Model file for the job. Use its own axes, mm. Face numbers are marked on the shaded views. A direction names the side the tool comes from. Give positions to 0.01 mm unless a question says otherwise; leave off trailing zeros. Loops run counter-clockwise (first coordinate to the right, second up) from the corner with the lowest first, then second, coordinate; pieces in that order, holes last. Notation, with made-up numbers: M -6.5,80.25 L 9.5,80.25 A21 ccw 9.5,116.25 Z; hole C 23,2 d2. An arc over 180 degrees is marked long. Use CSV: the item, a comma, the result in double quotes. Start each with the question number.
(1) Slice it at C-C on y = 46.5. List the corners of the cut face in (x, z).
(2) Two-plate mould, pull along Z, no slides. Class the marked faces 4, 5, 6 and 7: pulls with the +Z half, pulls with the -Z half, needs draft (parallel to the pull), parting line crosses it, or undercut.
(3) Wall check: line 1 along X through (y, z) = (62, -13.5); line 2 along Z through (x, y) = (12, 57); line 3 along Z through (x, y) = (-13, 58). Give the ranges that are in metal, low to high. Write a range as from..to.
(4) Slice it at A-A on z = -13. List the corners of the cut face in (x, y).
(5) Tool access for the marked faces 1, 2 and 3: list every direction of +Z, -Z, +X, -X, +Y, -Y with a clear straight run to the whole face (end or side of a thin tool).
(6) Flat gauge pins, fed straight in: P1, Ø5, axis at x = 12, y = 21, coming from the +Z side; P2, Ø2, axis at x = -8.5, y = 57, coming from the +Z side; P3, Ø8, axis at x = 4, z = 22, coming from the +Y side. Where does each tip first touch, or does it go through?
(7) Slice it at B-B on x = -6. List the corners of the cut face in (y, z).
(8) Slice it at D-D on z = 14. List the corners of the cut face in (x, y), and give its area (3 significant figures).
```python
from build123d import *

# Parameters (mm, degrees)
SKETCH1_R           = 17.5
BOSS_EXTRUDE1_DEPTH = 48
BOSS_EXTRUDE2_DEPTH = 15
BOSS_EXTRUDE3_DEPTH = 20


with BuildPart() as part:
    # Sketch1 → Boss-Extrude1 (new body)
    with BuildSketch(Plane(origin=(0, 0, 0), x_dir=(1, 0, 0), z_dir=(0, 1, 0))):
        Circle(SKETCH1_R)
    extrude(amount=BOSS_EXTRUDE1_DEPTH)

    # Sketch4 → Boss-Extrude2 (add)
    with BuildSketch(Plane.XZ):
        with BuildLine():
            Line((10.25, 23.304288773), (10.25, 16.761190292))
            ThreePointArc((10.25, 16.761190292), (10.701996736, 14.5776924), (11.983695652, 12.75307957))
            ThreePointArc((11.983695652, 12.75307957), (0, 17.5), (-11.983695652, 12.75307957))
            ThreePointArc((-11.983695652, 12.75307957), (-10.701996736, 14.5776924), (-10.25, 16.761190292))
            Line((-10.25, 16.761190292), (-10.25, 23.304288773))
            ThreePointArc((-10.25, 23.304288773), (-9.292662905, 26.079093189), (-6.827982425, 27.673265071))
            ThreePointArc((-6.827982425, 27.673265071), (0, 28.503174274), (6.827982425, 27.673265071))
            ThreePointArc((6.827982425, 27.673265071), (9.292662905, 26.079093189), (10.25, 23.304288773))
        make_face()
    extrude(amount=-BOSS_EXTRUDE2_DEPTH)

    # Sketch6 → Boss-Extrude3 (add)
    with BuildSketch(Plane(origin=(0, 48, 0), x_dir=(1, 0, 0), z_dir=(0, 1, 0))):
        with BuildLine():
            ThreePointArc((11.641553947, -1.685099566), (14.648632583, -1.806960077), (17.329910897, -0.440168758))
            ThreePointArc((17.329910897, -0.440168758), (17.3355, 0), (17.329910897, 0.440168758))
            ThreePointArc((17.329910897, 0.440168758), (14.648632583, 1.806960077), (11.641553947, 1.685099566))
            ThreePointArc((11.641553947, 1.685099566), (11.362069294, 3.044457292), (10.92443124, 4.361437941))
            ThreePointArc((10.92443124, 4.361437941), (13.589567986, 5.759442961), (15.228227462, 8.283758122))
            ThreePointArc((15.228227462, 8.283758122), (15.012983387, 8.66775), (14.788058703, 9.046152775))
            ThreePointArc((14.788058703, 9.046152775), (11.782607909, 8.889189622), (9.239331674, 7.280116005))
            ThreePointArc((9.239331674, 7.280116005), (8.317612002, 8.317612002), (7.280116005, 9.239331674))
            ThreePointArc((7.280116005, 9.239331674), (8.889189622, 11.782607909), (9.046152775, 14.788058703))
            ThreePointArc((9.046152775, 14.788058703), (8.66775, 15.012983387), (8.283758122, 15.228227462))
            ThreePointArc((8.283758122, 15.228227462), (5.759442961, 13.589567986), (4.361437941, 10.92443124))
            ThreePointArc((4.361437941, 10.92443124), (3.044457292, 11.362069294), (1.685099566, 11.641553947))
            ThreePointArc((1.685099566, 11.641553947), (1.806960077, 14.648632583), (0.440168758, 17.329910897))
            ThreePointArc((0.440168758, 17.329910897), (0, 17.3355), (-0.440168758, 17.329910897))
            ThreePointArc((-0.440168758, 17.329910897), (-1.806960077, 14.648632583), (-1.685099566, 11.641553947))
            ThreePointArc((-1.685099566, 11.641553947), (-3.044457292, 11.362069294), (-4.361437941, 10.92443124))
            ThreePointArc((-4.361437941, 10.92443124), (-5.759442961, 13.589567986), (-8.283758122, 15.228227462))
            ThreePointArc((-8.283758122, 15.228227462), (-8.66775, 15.012983387), (-9.046152775, 14.788058703))
            ThreePointArc((-9.046152775, 14.788058703), (-8.889189622, 11.782607909), (-7.280116005, 9.239331674))
            ThreePointArc((-7.280116005, 9.239331674), (-8.317612002, 8.317612002), (-9.239331674, 7.280116005))
            ThreePointArc((-9.239331674, 7.280116005), (-11.782607909, 8.889189622), (-14.788058703, 9.046152775))
            ThreePointArc((-14.788058703, 9.046152775), (-15.012983387, 8.66775), (-15.228227462, 8.283758122))
            ThreePointArc((-15.228227462, 8.283758122), (-13.589567986, 5.759442961), (-10.92443124, 4.361437941))
            ThreePointArc((-10.92443124, 4.361437941), (-11.362069294, 3.044457292), (-11.641553947, 1.685099566))
            ThreePointArc((-11.641553947, 1.685099566), (-14.648632583, 1.806960077), (-17.329910897, 0.440168758))
            ThreePointArc((-17.329910897, 0.440168758), (-17.3355, 0), (-17.329910897, -0.440168758))
            ThreePointArc((-17.329910897, -0.440168758), (-14.648632583, -1.806960077), (-11.641553947, -1.685099566))
            ThreePointArc((-11.641553947, -1.685099566), (-11.362069294, -3.044457292), (-10.92443124, -4.361437941))
            ThreePointArc((-10.92443124, -4.361437941), (-13.589567986, -5.759442961), (-15.228227462, -8.283758122))
            ThreePointArc((-15.228227462, -8.283758122), (-15.012983387, -8.66775), (-14.788058703, -9.046152775))
            ThreePointArc((-14.788058703, -9.046152775), (-11.782607909, -8.889189622), (-9.239331674, -7.280116005))
            ThreePointArc((-9.239331674, -7.280116005), (-8.317612002, -8.317612002), (-7.280116005, -9.239331674))
            ThreePointArc((-7.280116005, -9.239331674), (-8.889189622, -11.782607909), (-9.046152775, -14.788058703))
            ThreePointArc((-9.046152775, -14.788058703), (-8.66775, -15.012983387), (-8.283758122, -15.228227462))
            ThreePointArc((-8.283758122, -15.228227462), (-5.759442961, -13.589567986), (-4.361437941, -10.92443124))
            ThreePointArc((-4.361437941, -10.92443124), (-3.044457292, -11.362069294), (-1.685099566, -11.641553947))
            ThreePointArc((-1.685099566, -11.641553947), (-1.806960077, -14.648632583), (-0.440168758, -17.329910897))
            ThreePointArc((-0.440168758, -17.329910897), (0, -17.3355), (0.440168758, -17.329910897))
            ThreePointArc((0.440168758, -17.329910897), (1.806960077, -14.648632583), (1.685099566, -11.641553947))
            ThreePointArc((1.685099566, -11.641553947), (3.044457292, -11.362069294), (4.361437941, -10.92443124))
            ThreePointArc((4.361437941, -10.92443124), (5.759442961, -13.589567986), (8.283758122, -15.228227462))
            ThreePointArc((8.283758122, -15.228227462), (8.66775, -15.012983387), (9.046152775, -14.788058703))
            ThreePointArc((9.046152775, -14.788058703), (8.889189622, -11.782607909), (7.280116005, -9.239331674))
            ThreePointArc((7.280116005, -9.239331674), (8.317612002, -8.317612002), (9.239331674, -7.280116005))
            ThreePointArc((9.239331674, -7.280116005), (11.782607909, -8.889189622), (14.788058703, -9.046152775))
            ThreePointArc((14.788058703, -9.046152775), (15.012983387, -8.66775), (15.228227462, -8.283758122))
            ThreePointArc((15.228227462, -8.283758122), (13.589567986, -5.759442961), (10.92443124, -4.361437941))
            ThreePointArc((10.92443124, -4.361437941), (11.362069294, -3.044457292), (11.641553947, -1.685099566))
        make_face()
    extrude(amount=BOSS_EXTRUDE3_DEPTH)


solid = part.part
```
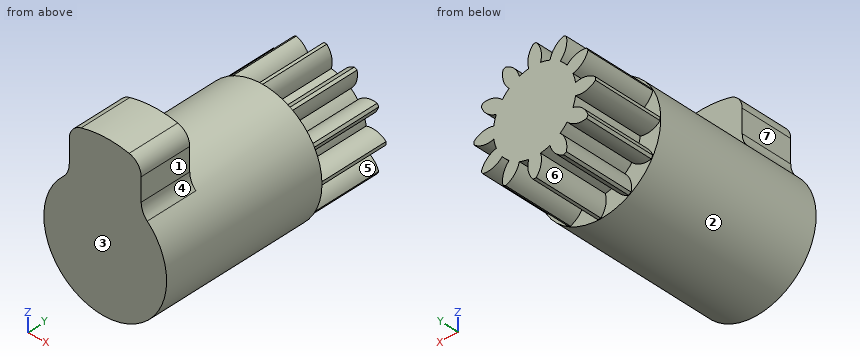
Reply:
1,outline,"C 0,0 d35"
2,face 4,"pulls with the +Z half"
2,face 5,"undercut"
2,face 6,"undercut"
2,face 7,"needs draft"
3,line 1,"x = -9.17..-5.68, -1.94..1.94, 5.68..9.17"
3,line 2,"z = -8.95..-4.72, -1.78..1.78, 4.72..8.95"
3,line 3,"z = -9.14..-5.29, -1.93..1.93, 5.29..9.14"
4,outline,"M -11.72,0 L 11.72,0 L 11.72,48 L 9.14,48 L 9.14,68 L 5.29,68 L 5.29,48 L 1.93,48 L 1.93,68 L -1.93,68 L -1.93,48 L -5.29,48 L -5.29,68 L -9.14,68 L -9.14,48 L -11.72,48 Z"
5,face 1,"+Z, +X, +Y, -Y"
5,face 2,"+Y"
5,face 3,"+Z, -Z, +X, -X, -Y"
6,P1,"stops at z = 14.7"
6,P2,"stops at z = 15.23"
6,P3,"stops at y = 15"
7,outline,"M 0,-16.44 L 48,-16.44 L 48,-13.84 L 68,-13.84 L 68,13.84 L 48,13.84 L 48,16.44 L 15,16.44 L 15,27.86 L 0,27.86 Z"
8,outline,"M -10.99,0 L 10.99,0 L 10.99,15 L 10.5,15 L 10.5,48 L 9.15,48 L 9.15,68 L 6.17,68 L 6.17,48 L 1.91,48 L 1.91,68 L -1.91,68 L -1.91,48 L -6.17,48 L -6.17,68 L -9.15,68 L -9.15,48 L -10.5,48 L -10.5,15 L -10.99,15 Z"
8,area,"1,220 mm^2"
